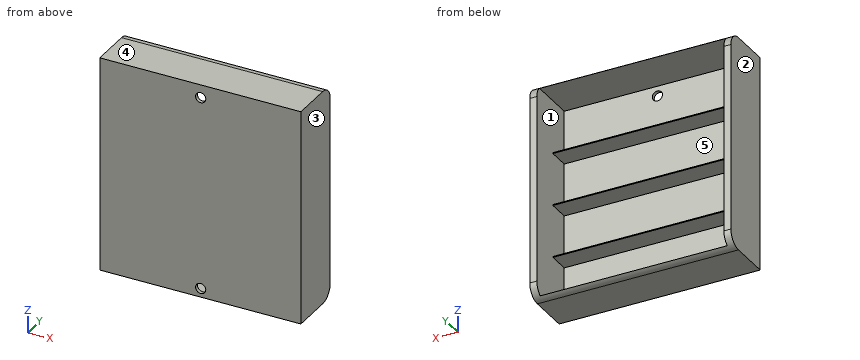
```python
from build123d import *

# Parameters (mm, degrees)
SKETCH1_W                  = 57.2
SKETCH1_H                  = 61.3
BOSS_EXTRUDE1_DEPTH        = 15.5
F_2_9_2_9_DIAMETER_HOLE1_D = 2.9
SKETCH4_W                  = 53.2
SKETCH4_H                  = 59.75
CUT_EXTRUDE1_DEPTH         = 14.5
FILLET4_R                  = 4
SKETCH5_W                  = 53.2
SKETCH5_H                  = 0.25
BOSS_EXTRUDE2_DEPTH        = 6
LPATTERN1_COUNT            = 3
LPATTERN1_PITCH            = 15


with BuildPart() as part:
    # Sketch1 → Boss-Extrude1 (new body)
    with BuildSketch(Plane(origin=(0, 0, 0), x_dir=(1, 0, 0), z_dir=(0, 1, 0))):
        with Locations((28.6, 30.65)):
            Rectangle(SKETCH1_W, SKETCH1_H)
    extrude(amount=BOSS_EXTRUDE1_DEPTH)

    # Ø2.9 (2.9) Diameter Hole1 (through all)
    with Locations(Plane(origin=(0, 15.5, 0), x_dir=(-1, 0, 0), z_dir=(0, 1, 0))):
        with Locations((-28.7, -58.8), (-28.7, -3.7)):
            Hole(F_2_9_2_9_DIAMETER_HOLE1_D / 2)

    # Sketch4 → Cut-Extrude1 (cut)
    with BuildSketch(Plane(origin=(0, 15.5, 0), x_dir=(1, 0, 0), z_dir=(0, 1, 0))):
        with Locations((28.6, 30.775)):
            Rectangle(SKETCH4_W, SKETCH4_H)
    extrude(amount=-CUT_EXTRUDE1_DEPTH, mode=Mode.SUBTRACT)

    # Fillet4
    # the kernel refuses this fillet: 4 mm, written as the material it takes off along each edge
    with BuildSketch(Plane(origin=(-10, 15.5, 0), x_dir=(0, -1, 0), z_dir=(1, 0, 0))) as fillet4_piece_1:
        with BuildLine():
            CenterArc((FILLET4_R, FILLET4_R), FILLET4_R, 180, 90)
            Line((0, FILLET4_R), (0, 0))
            Line((0, 0), (FILLET4_R, 0))
        make_face()
    extrude(amount=77.2, mode=Mode.SUBTRACT)
    with BuildSketch(Plane(origin=(67.2, 15.5, -61.3), x_dir=(0, 0, 1), z_dir=(-1, 0, 0))) as fillet4_piece_2:
        with BuildLine():
            CenterArc((FILLET4_R, -FILLET4_R), FILLET4_R, 90, 90)
            Line((0, -FILLET4_R), (0, 0))
            Line((0, 0), (FILLET4_R, 0))
        make_face()
    extrude(amount=77.2, mode=Mode.SUBTRACT)

    # Sketch5 → Boss-Extrude2 (add)
    with BuildSketch(Plane(origin=(0, 1, 0), x_dir=(1, 0, 0), z_dir=(0, 1, 0))):
        with Locations((28.6, 16.025)):
            Rectangle(SKETCH5_W, SKETCH5_H)
    boss_extrude2 = extrude(amount=BOSS_EXTRUDE2_DEPTH)

    # LPattern1: Boss-Extrude2 ×3
    with Locations(*[(0, 0, -i * LPATTERN1_PITCH) for i in range(1, LPATTERN1_COUNT)]):
        add(boss_extrude2)


solid = part.part
```
Work out the finished part from the listing and answer in its coordinate system (mm). Face numbers are marked on the shaded views. A direction names the side the tool comes from. Round coordinates to 2 decimals unless told otherwise and drop trailing zeros. Order: outer loops, then holes, each group sorted by start corner. A loop starts at its lowest first (then second) coordinate and runs counter-clockwise, first axis right, second up.
Q1. A cutting plane is placed at A-A, the plane y = 9. Determine the outline of the cut face in (x, z).
Solution:
outline: (0, -61.3) - (57.2, -61.3) - (57.2, 0) - (0, 0) - close; hole (2, -60.65) - (55.2, -60.65) - (55.2, -0.9) - (2, -0.9) - close
Q2. Given pin 1 Ø6.5 at (x, y) = (37.5, 10.5) entering from +Z; pin 2 Ø12 at (x, z) = (32.5, -23) entering from +Y; pin 3 Ø16 at (x, z) = (25.5, -50) entering from +Y, each flat-ended and moving along its own axis, determine where each tip first touches the part or whether it passes through.
Solution:
pin 1: stops at z = 0
pin 2: stops at y = 1
pin 3: stops at y = 7
Q3. A cutting plane is placed at B-B, the plane x = 28.7. Determine the outline of the cut face in (y, z).
Solution:
outline: (0, -61.3) - (11.5, -61.3) arc R4 ccw to (13.69, -60.65) - (1, -60.65) - (1, -60.25) - (0, -60.25) - close; (0, -57.35) - (1, -57.35) - (1, -46.15) - (7, -46.15) - (7, -45.9) - (1, -45.9) - (1, -31.15) - (7, -31.15) - (7, -30.9) - (1, -30.9) - (1, -16.15) - (7, -16.15) - (7, -15.9) - (1, -15.9) - (1, -5.15) - (0, -5.15) - close; (0, -2.25) - (1, -2.25) - (1, -0.9) - (14.03, -0.9) arc R4 ccw to (11.5, 0) - (0, 0) - close
Q4. Find the intervals of material crossed by line 1 along Z through (x, y) = (28, 3.25); line 2 along Z through (x, y) = (28.7, 0.55); line 3 along X through (y, z) = (12, -27.5), in increasing order.
Solution:
line 1: z = -61.3 to -60.65, -46.15 to -45.9, -31.15 to -30.9, -16.15 to -15.9, -0.9 to 0
line 2: z = -61.3 to -60.25, -57.35 to -5.15, -2.25 to 0
line 3: x = 0 to 2, 55.2 to 57.2
Q5. A tool of negligible diameter and unlimited length cuts with its end or side. For the marked faces 1 and 2, from which of +Z, -Z, +X, -X, +Y, -Y can it reach the whole face along a straight path? Write none if from no direction.
Solution:
face 1: +Y
face 2: +Z, -Z, -X, +Y, -Y
Q6. The mould has two halves that part along X. Classify the marked faces 3, 4 and 5: pulls with the +X half, pulls with the -X half, needs draft (parallel to the pull), parting line crosses it, or undercut.
Solution:
face 3: pulls with the +X half
face 4: needs draft
face 5: undercut
Q7. A cutting plane is placed at C-C, the plane y = 4.75. Determine the outline of the cut face in (x, z), then the cut area to 3 significant figures.
Solution:
outline: (0, -61.3) - (57.2, -61.3) - (57.2, 0) - (0, 0) - close; hole (2, -60.65) - (55.2, -60.65) - (55.2, -46.15) - (2, -46.15) - close; hole (2, -45.9) - (55.2, -45.9) - (55.2, -31.15) - (2, -31.15) - close; hole (2, -30.9) - (55.2, -30.9) - (55.2, -16.15) - (2, -16.15) - close; hole (2, -15.9) - (55.2, -15.9) - (55.2, -0.9) - (2, -0.9) - close
area: 368 mm2
Q8. A cutting plane is placed at D-D, the plane z = -58.8. Determine the outline of the cut face in (x, y), then the cut area to 3 significant figures.
Solution:
outline: (0, 0) - (27.25, 0) - (27.25, 1) - (2, 1) - (2, 15.21) - (0, 15.21) - close; (30.15, 0) - (57.2, 0) - (57.2, 15.21) - (55.2, 15.21) - (55.2, 1) - (30.15, 1) - close
area: 111 mm2
